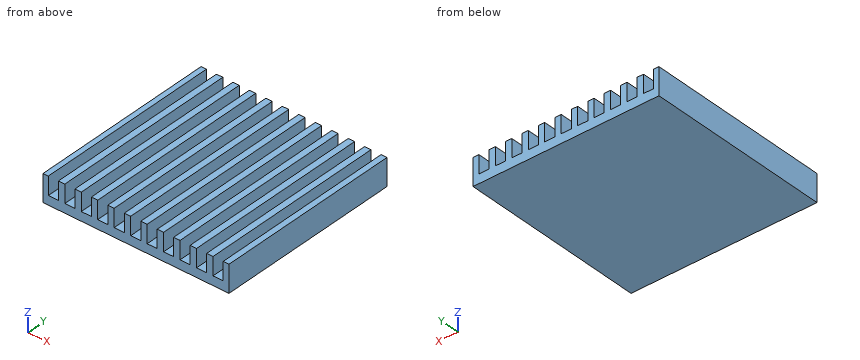
```python
from build123d import *

# Parameters (mm, degrees)
SKETCH_1_W          = 35
SKETCH_1_H          = 35
EXTRUDE_1_DEPTH     = 5.1
SKETCH_2_W          = 1.9
SKETCH_2_H          = 3.4
CUT_EXTRUDE_1_DEPTH = 50.759521702


with BuildPart() as part:
    # 草图1 → 凸台-拉伸1 (new body)
    with BuildSketch(Plane.XY):
        with Locations((17.5, -17.5)):
            Rectangle(SKETCH_1_W, SKETCH_1_H)
    extrude(amount=EXTRUDE_1_DEPTH)

    # 草图2 → 切除-拉伸1 (cut, through all)
    with BuildSketch(Plane.XZ.offset(35)):
        with Locations((1.95, 3.4)):
            Rectangle(SKETCH_2_W, SKETCH_2_H)
        with Locations((5.05, 3.4)):
            Rectangle(SKETCH_2_W, SKETCH_2_H)
        with Locations((8.15, 3.4)):
            Rectangle(SKETCH_2_W, SKETCH_2_H)
        with Locations((11.25, 3.4)):
            Rectangle(SKETCH_2_W, SKETCH_2_H)
        with Locations((14.35, 3.4)):
            Rectangle(SKETCH_2_W, SKETCH_2_H)
        with Locations((17.45, 3.4)):
            Rectangle(SKETCH_2_W, SKETCH_2_H)
        with Locations((20.55, 3.4)):
            Rectangle(SKETCH_2_W, SKETCH_2_H)
        with Locations((23.65, 3.4)):
            Rectangle(SKETCH_2_W, SKETCH_2_H)
        with Locations((26.75, 3.4)):
            Rectangle(SKETCH_2_W, SKETCH_2_H)
        with Locations((29.85, 3.4)):
            Rectangle(SKETCH_2_W, SKETCH_2_H)
        with Locations((32.95, 3.4)):
            Rectangle(SKETCH_2_W, SKETCH_2_H)
    extrude(amount=-CUT_EXTRUDE_1_DEPTH, mode=Mode.SUBTRACT)


solid = part.part
```
Model file for the job. Use its own axes, mm. Give positions to 0.01 mm unless a question says otherwise; leave off trailing zeros. Write each loop counter-clockwise with the first axis right and the second up, starting at its lowest first coordinate (ties: lowest second). Pieces come first, ordered by that corner, then holes. Notation, with made-up numbers: (-25, -10) - (-1, -10) arc R33 cw to (-1, 26) - close; hole circle Ø4 at (47, 35). An arc over 180 degrees is marked (long way). One line per question, with ' | ' between items. Start each with the question number.
(1) Wall check: line 1 along Z through (x, y) = (2.5, -6). Give the ranges that are in metal, low to high. Write a range as from..to.
(2) Slice it at A-A on z = 2.25. Give the number of separate pieces and of enclosed holes in the cut face, plus the area to 4 significant figures.
(3) Pin check, flat tip, straight feed: P1, Ø1, axis at x = 14.5, y = -14.5, coming from the +Z side. Stop position of the tip, or through.
(4) Slice it at B-B on x = 4.5. Write the cut outline in (y, z).
Results below:
1) line 1: 0..1.7
2) separate pieces: 12 | enclosed holes: 0 | area: 493.5 mm^2
3) P1: z = 1.7
4) outline: (-35, 0) - (0, 0) - (0, 1.7) - (-35, 1.7) - close
